Check sheet for the modelled part. Datum: model origin and axes. Units: mm. A direction names the side the tool comes from. Round coordinates to 2 decimals unless told otherwise and drop trailing zeros. Order: outer loops, then holes, each group sorted by start corner. A loop starts at its lowest first (then second) coordinate and runs counter-clockwise, first axis right, second up. Notation, with made-up numbers: (19.5, -34.5) -> (38.5, -34.5) arc R26 ccw to (38.5, -8.5) -> close; hole circle Ø3 at (76, 86). An arc over 180 degrees is marked (long way). Answer in a Markdown table with one row per item.
Autodesk Inventor part; units mm, degrees
ref_plane "YZ Plane" through (0, 0, 0) normal (1, 0, 0) x (0, 1, 0)
ref_plane "XZ Plane" through (0, 0, 0) normal (0, 1, 0) x (-1, 0, 0)
ref_plane "XY Plane" through (0, 0, 0) normal (0, 0, 1) x (1, 0, 0)
sketch "Boceto1" plane through (0, 0, 0) normal (0, 0, 1) x (1, 0, 0)
  line L0 (0, 0) -> (0, 0.3)
  line L1 (1.35, 0.9) -> (1.35, 11.3)
  line L2 (1.35, 11.3) -> (0, 0.3)
  line L3 (3.75, 0.9) -> (3.75, 11.3)
  line L4 (3.75, 11.3) -> (5.1, 0.3)
  line L5 (5.1, 0) -> (5.1, 0.3)
  line L6 (1.35, 0.9) -> (3.75, 0.9)
  line L7 (3.75, 0.6) -> (1.35, 0.6)
  line L8 (3.75, 0.6) -> (3.75, 0)
  line L9 (1.35, 0.6) -> (1.35, 0)
  line L10 (0, 0) -> (1.35, 0)
  line L11 (3.75, 0) -> (5.1, 0)
  line L12 (1.35, 11.3) -> (1.85, 11.3)
  line L13 (1.85, 11.3) -> (1.85, 0.9)
  line L14 (3.75, 11.3) -> (3.25, 11.3)
  line L15 (3.25, 11.3) -> (3.25, 0.9)
extrude "Extrusión1" add sketch "Boceto1" along normal blind 1.2 contours L0 L2 L1 L6 L3 L4 L5 L11 L8 L7 L9 L10
sketch "Boceto2" plane through (1.35, 0.9, 0) normal (0, 1, 0) x (1, 0, 0)
  line L0 (2.55, 0) -> (-0.15, 0)
  line L1 (-0.15, 0) -> (-0.15, -1.2)
  line L2 (-0.15, -1.2) -> (2.55, -1.2)
  line L3 (2.55, -1.2) -> (2.55, 0)
  line L4 (0, 0) -> (0, -1.2)
  line L5 (2.4, 0) -> (2.4, -1.2)
  line L6 (-0.15, -1.2) -> (-1.35, -1.2)
  line L7 (-1.35, -1.2) -> (-1.35, 0)
  line L8 (-1.35, 0) -> (-0.15, 0)
  line L9 (-0.15, 0) -> (-0.15, -0.15)
  line L10 (-0.15, -0.15) -> (-1.35, -0.15)
  line L11 (-1.35, -1.05) -> (-0.15, -1.05)
  line L12 (2.55, -1.2) -> (3.75, -1.2)
  line L13 (3.75, -1.2) -> (3.75, 0)
  line L14 (3.75, 0) -> (2.55, 0)
  line L15 (2.55, -0.15) -> (3.75, -0.15)
  line L16 (3.75, -1.05) -> (2.55, -1.05)
  line L17 (2.4, 0) -> (1.9, 0)
  line L18 (1.9, 0) -> (1.9, -0.15)
  line L19 (0, 0) -> (0.5, 0)
  line L20 (0.5, 0) -> (0.5, -0.15)
  arc A0 (2.3906, -1.2) -> (1.9, -0.3753) centre (1.2, -1.35) ccw
  line L21 (0, -1.2) -> (0.0094, -1.2)
  line L22 (0.5, -0.15) -> (0.5, -0.3753)
  line L23 (1.9, -0.15) -> (1.9, -0.3753)
  line L24 (2.4, -1.2) -> (2.3906, -1.2)
  arc A1 (0.5, -0.3753) -> (0.0094, -1.2) centre (1.2, -1.35) ccw
  line L25 (0, 0) -> (-1.35, 0)
  line L26 (-1.35, 0) -> (-1.35, -1.2)
  line L27 (0, -1.2) -> (-1.35, -1.2)
  line L28 (0, 0) -> (0, -1.2)
  line L29 (3.75, 0) -> (2.4, 0)
  line L30 (2.4, 0) -> (2.4, -1.2)
  line L31 (3.75, -1.2) -> (2.4, -1.2)
  line L32 (3.75, 0) -> (3.75, -1.2)
  line L33 (2.4, 0) -> (0, 0)
  line L34 (0, 0) -> (0, -1.2)
  line L35 (2.4, -1.2) -> (0, -1.2)
  line L36 (2.4, 0) -> (2.4, -1.2)
extrude "Extrusión2" cut sketch "Boceto2" along normal blind 12 contours L15 L13 L16 L3 | L1 L11 L7 L10
sketch "Boceto3" plane through (1.35, 0.9, 0) normal (0, 1, 0) x (1, 0, 0)
  line L0 (2.55, 0) -> (-0.15, 0)
  line L1 (-0.15, 0) -> (-0.15, -1.2)
  line L2 (-0.15, -1.2) -> (2.55, -1.2)
  line L3 (2.55, -1.2) -> (2.55, 0)
  line L4 (0, 0) -> (0, -1.2)
  line L5 (2.4, 0) -> (2.4, -1.2)
  line L6 (-0.15, -1.2) -> (-1.35, -1.2)
  line L7 (-1.35, -1.2) -> (-1.35, 0)
  line L8 (-1.35, 0) -> (-0.15, 0)
  line L9 (-0.15, 0) -> (-0.15, -0.15)
  line L10 (-0.15, -0.15) -> (-1.35, -0.15)
  line L11 (-1.35, -1.05) -> (-0.15, -1.05)
  line L12 (2.55, -1.2) -> (3.75, -1.2)
  line L13 (3.75, -1.2) -> (3.75, 0)
  line L14 (3.75, 0) -> (2.55, 0)
  line L15 (2.55, -0.15) -> (3.75, -0.15)
  line L16 (3.75, -1.05) -> (2.55, -1.05)
  line L17 (2.4, 0) -> (1.9, 0)
  line L18 (1.9, 0) -> (1.9, -0.15)
  line L19 (0, 0) -> (0.5, 0)
  line L20 (0.5, 0) -> (0.5, -0.15)
  arc A0 (2.3906, -1.2) -> (1.9, -0.3753) centre (1.2, -1.35) ccw
  line L21 (0, -1.2) -> (0.0094, -1.2)
  line L22 (0.5, -0.15) -> (0.5, -0.3753)
  line L23 (1.9, -0.15) -> (1.9, -0.3753)
  line L24 (2.4, -1.2) -> (2.3906, -1.2)
  arc A1 (0.5, -0.3753) -> (0.0094, -1.2) centre (1.2, -1.35) ccw
  line L25 (0, 0) -> (-1.35, 0)
  line L26 (-1.35, 0) -> (-1.35, -1.2)
  line L27 (0, -1.2) -> (-1.35, -1.2)
  line L28 (0, 0) -> (0, -1.2)
  line L29 (3.75, 0) -> (2.4, 0)
  line L30 (2.4, 0) -> (2.4, -1.2)
  line L31 (3.75, -1.2) -> (2.4, -1.2)
  line L32 (3.75, 0) -> (3.75, -1.2)
  line L33 (2.4, 0) -> (0, 0)
  line L34 (0, 0) -> (0, -1.2)
  line L35 (2.4, -1.2) -> (0, -1.2)
  line L36 (2.4, 0) -> (2.4, -1.2)
extrude "Extrusión3" add sketch "Boceto3" along normal blind 10.4 contours L5 L2 A0 L23 L18 L0 | L20 L22 A1 L2 L4 L0
sketch "Boceto4" plane through (1.35, 11.3, 0) normal (0, 1, 0) x (1, 0, 0)
  line L0 (0, 0) -> (0, -1.2)
  line L1 (0, -1.2) -> (0.0094, -1.2)
  arc A0 (0.5, -0.3753) -> (0.0094, -1.2) centre (1.2, -1.35) ccw
  line L2 (0.5, -0.3753) -> (0.5, 0)
  line L3 (0.5, 0) -> (0, 0)
  line L4 (2.4, 0) -> (1.9, 0)
  line L5 (1.9, 0) -> (1.9, -0.3753)
  arc A1 (2.3906, -1.2) -> (1.9, -0.3753) centre (1.2, -1.35) ccw
  line L6 (2.3906, -1.2) -> (2.4, -1.2)
  line L7 (2.4, 0) -> (2.4, -1.2)
  line L8 (2.55, 0) -> (-0.15, 0)
  line L9 (-0.15, 0) -> (-0.15, -1.2)
  line L10 (-0.15, -1.2) -> (2.55, -1.2)
  line L11 (2.55, -1.2) -> (2.55, 0)
  line L12 (0, 0) -> (0, -1.2)
  line L13 (2.4, 0) -> (2.4, -1.2)
  line L14 (-0.15, -1.2) -> (-1.35, -1.2)
  line L15 (-1.35, -1.2) -> (-1.35, 0)
  line L16 (-1.35, 0) -> (-0.15, 0)
  line L17 (-0.15, 0) -> (-0.15, -0.15)
  line L18 (-0.15, -0.15) -> (-1.35, -0.15)
  line L19 (-1.35, -1.05) -> (-0.15, -1.05)
  line L20 (2.55, -1.2) -> (3.75, -1.2)
  line L21 (3.75, -1.2) -> (3.75, 0)
  line L22 (3.75, 0) -> (2.55, 0)
  line L23 (2.55, -0.15) -> (3.75, -0.15)
  line L24 (3.75, -1.05) -> (2.55, -1.05)
  line L25 (2.4, 0) -> (1.9, 0)
  line L26 (1.9, 0) -> (1.9, -0.15)
  line L27 (0, 0) -> (0.5, 0)
  line L28 (0.5, 0) -> (0.5, -0.15)
  arc A2 (2.3906, -1.2) -> (1.9, -0.3753) centre (1.2, -1.35) ccw
  line L29 (0, -1.2) -> (0.0094, -1.2)
  line L30 (0.5, -0.15) -> (0.5, -0.3753)
  line L31 (1.9, -0.15) -> (1.9, -0.3753)
  line L32 (2.4, -1.2) -> (2.3906, -1.2)
  arc A3 (0.5, -0.3753) -> (0.0094, -1.2) centre (1.2, -1.35) ccw
  point P0 (-1.35, 0)
extrude "Extrusión4" add sketch "Boceto4" against normal blind 10.4 contours L0 L10 L9 L8 | L8 L11 L10 L7
sketch "Boceto5" plane through (1.35, 11.3, 0) normal (0, 1, 0) x (1, 0, 0)
  line L0 (2.55, 0) -> (-0.15, 0)
  line L1 (-0.15, 0) -> (-0.15, -1.2)
  line L2 (-0.15, -1.2) -> (2.55, -1.2)
  line L3 (0, 0) -> (0, -1.2)
  line L4 (2.4, 0) -> (2.4, -1.2)
  line L5 (0, -1.2) -> (0.0094, -1.2)
  line L6 (0.5, -0.15) -> (0.5, -0.3753)
  line L7 (0, 0) -> (0.5, 0)
  line L8 (0.5, 0) -> (0.5, -0.15)
  arc A0 (0.5, -0.3753) -> (0.0094, -1.2) centre (1.2, -1.35) ccw
  line L9 (2.4, -1.2) -> (0, -1.2)
  line L10 (2.4, 0) -> (0, 0)
  line L11 (1.9, 0) -> (1.9, -0.15)
  line L12 (2.4, 0) -> (1.9, 0)
  line L13 (-0.15, -1.2) -> (-1.35, -1.2)
  line L14 (-1.35, -1.2) -> (-1.35, 0)
  line L15 (-1.35, 0) -> (-0.15, 0)
  line L16 (-0.15, 0) -> (-0.15, -0.15)
  line L17 (0, 0) -> (0, -1.2)
  line L18 (0, 0) -> (-1.35, 0)
  line L19 (-0.15, -0.15) -> (-1.35, -0.15)
  line L20 (-1.35, -1.05) -> (-0.15, -1.05)
  line L21 (-1.35, 0) -> (-1.35, -1.2)
  line L22 (0, -1.2) -> (-1.35, -1.2)
  line L23 (0, 0) -> (0, -1.2)
  line L24 (2.55, -1.2) -> (2.55, 0)
  line L25 (2.55, -1.2) -> (3.75, -1.2)
  line L26 (3.75, -1.2) -> (3.75, 0)
  line L27 (3.75, 0) -> (2.55, 0)
  line L28 (2.55, -0.15) -> (3.75, -0.15)
  line L29 (3.75, -1.05) -> (2.55, -1.05)
  line L30 (1.9, -0.15) -> (1.9, -0.3753)
  arc A1 (2.3906, -1.2) -> (1.9, -0.3753) centre (1.2, -1.35) ccw
  line L31 (2.4, -1.2) -> (2.3906, -1.2)
  line L32 (2.4, 0) -> (2.4, -1.2)
  line L33 (2.4, 0) -> (2.4, -1.2)
  line L34 (3.75, -1.2) -> (2.4, -1.2)
  line L35 (3.75, 0) -> (3.75, -1.2)
  line L36 (3.75, 0) -> (2.4, 0)
extrude "Extrusión5" cut sketch "Boceto5" against normal blind 11 contours L28 L26 L29 L24 | L1 L20 L14 L19
sketch "Boceto6" plane through (1.35, 0.3, 0) normal (0, 1, 0) x (1, 0, 0)
  line L0 (2.55, 0) -> (-0.15, 0)
  line L1 (-0.15, 0) -> (-0.15, -1.2)
  line L2 (-0.15, -1.2) -> (2.55, -1.2)
  line L3 (2.55, -1.2) -> (2.55, 0)
  line L4 (0, 0) -> (0, -1.2)
  line L5 (2.4, 0) -> (2.4, -1.2)
  line L6 (-0.15, -1.2) -> (-1.35, -1.2)
  line L7 (-1.35, -1.2) -> (-1.35, 0)
  line L8 (-1.35, 0) -> (-0.15, 0)
  line L9 (-0.15, 0) -> (-0.15, -0.15)
  line L10 (-0.15, -0.15) -> (-1.35, -0.15)
  line L11 (-1.35, -1.05) -> (-0.15, -1.05)
  line L12 (2.55, -1.2) -> (3.75, -1.2)
  line L13 (3.75, -1.2) -> (3.75, 0)
  line L14 (3.75, 0) -> (2.55, 0)
  line L15 (2.55, -0.15) -> (3.75, -0.15)
  line L16 (3.75, -1.05) -> (2.55, -1.05)
  line L17 (2.4, 0) -> (1.9, 0)
  line L18 (1.9, 0) -> (1.9, -0.15)
  line L19 (0, 0) -> (0.5, 0)
  line L20 (0.5, 0) -> (0.5, -0.15)
  arc A0 (2.3906, -1.2) -> (1.9, -0.3753) centre (1.2, -1.35) ccw
  line L21 (0, -1.2) -> (0.0094, -1.2)
  line L22 (0.5, -0.15) -> (0.5, -0.3753)
  line L23 (1.9, -0.15) -> (1.9, -0.3753)
  line L24 (2.4, -1.2) -> (2.3906, -1.2)
  arc A1 (0.5, -0.3753) -> (0.0094, -1.2) centre (1.2, -1.35) ccw
  circle A2 centre (2.75, -0.6) radius 0.15
  circle A3 centre (3.35, -0.6) radius 0.15
  circle A4 centre (-0.35, -0.6) radius 0.15
  circle A5 centre (-0.95, -0.6) radius 0.15
  line L25 (-1.35, 0) -> (-1.35, -0.15)
  line L26 (-1.35, -0.15) -> (-1.35, -1.05)
  line L27 (-1.35, -1.05) -> (-1.35, -1.2)
extrude "Extrusión6" cut sketch "Boceto6" against normal blind 10 contours A2 | A3 | A4 | A5
sketch "Boceto7" plane through (0, 0, 1.2) normal (0, 0, 1) x (1, 0, 0)
  line L0 (0, 0) -> (1.35, 0)
  line L1 (1.35, 0) -> (1.3594, 6.1)
  line L2 (1.3594, 0.9) -> (1.3594, 11.3)
  line L3 (1.3594, 6.1) -> (7.7947, 6.0901)
  line L4 (7.7947, 6.0901) -> (7.8047, 12.5901)
  line L5 (7.8047, 12.5901) -> (-2.1953, 12.6055)
  line L6 (-2.1953, 12.6055) -> (-2.2053, 6.1055)
  line L7 (-2.2053, 6.1055) -> (1.3594, 6.1)
  dimension "d12" = 6.1
  dimension "d13" = 6.5
  dimension "d14" = 10
extrude "Extrusión7" cut sketch "Boceto7" against normal blind 10
sketch "Boceto8" plane through (0, 0, 1.2) normal (0, 0, 1) x (1, 0, 0)
  line L0 (1.2, 6.1002) -> (1.2, 0.3)
  line L1 (3.9, 6.0961) -> (3.9, 0.3)
  line L2 (0, 0.3) -> (0, 0)
  line L3 (5.1, 0) -> (5.1, 0.3)
  line L4 (0, 0.3) -> (1.2, 6.1002)
  line L5 (1.2, 6.873) -> (1.2, 6.1002)
  line L6 (0, 0.3) -> (-0.3806, 0.3)
  line L7 (-0.3806, 0.3) -> (-0.3806, 6.873)
  line L8 (-0.3806, 6.873) -> (1.2, 6.873)
  line L9 (3.25, 0.9) -> (1.85, 0.9)
  line L10 (2.55, 0.9) -> (2.55, 4.8471)
  line L11 (3.9, 6.1002) -> (3.9, 0.3)
  line L12 (5.1, 0.3) -> (5.1, 0)
  line L13 (5.1, 0.3) -> (3.9, 6.1002)
  line L14 (3.9, 6.873) -> (3.9, 6.1002)
  line L15 (5.1, 0.3) -> (5.4806, 0.3)
  line L16 (5.4806, 0.3) -> (5.4806, 6.873)
  line L17 (5.4806, 6.873) -> (3.9, 6.873)
extrude "Extrusión8" cut sketch "Boceto8" against normal blind 10
sketch "Boceto9" plane through (0, 0, 1.2) normal (0, 0, 1) x (1, 0, 0)
  line L0 (0, 0) -> (0, 0.3)
  line L1 (1.35, 0.9) -> (1.35, 6.1)
  line L2 (1.2, 6.1) -> (0, 0.3)
  line L3 (3.75, 0.9) -> (3.75, 6.1)
  line L4 (3.9, 6.1) -> (5.1, 0.3)
  line L5 (5.1, 0) -> (5.1, 0.3)
  line L6 (1.35, 0.9) -> (3.75, 0.9)
  line L7 (3.75, 0.6) -> (1.35, 0.6)
  line L8 (3.75, 0.6) -> (3.75, 0)
  line L9 (1.35, 0.6) -> (1.35, 0)
  line L10 (0, 0) -> (1.35, 0)
  line L11 (3.75, 0) -> (5.1, 0)
  line L12 (1.85, 6.1) -> (1.85, 0.9)
  line L13 (3.25, 6.1) -> (3.25, 0.9)
  line L14 (1.2, 6.1) -> (1.85, 6.1)
  line L15 (3.25, 6.1) -> (3.75, 6.1)
  line L16 (1.35, 6.1) -> (1.2, 6.1)
  line L17 (3.75, 6.1) -> (3.9, 6.1)
  circle A0 centre (1.0336, 4) radius 0.15
  circle A1 centre (1.0336, 3.1) radius 0.15
  circle A2 centre (4.0664, 4) radius 0.15
  circle A3 centre (4.0664, 3.1) radius 0.15
  line L18 (1.35, 0.6) -> (3.75, 0.6)
  point P0 (0, 0)
extrude "Extrusión9" cut sketch "Boceto9" against normal blind 0.5 contours A0 | A1 | A2 | A3
properties part number "learnbotEncajeBateria"
(1) Section check D-D on x = 1.05. Record the boundary of the cut face in (y, z).
Solutions:
| item | result |
|---|---|
| outline | (0, 0) -> (5.38, 0) -> (5.38, 0.15) -> (0.3, 0.15) -> (0.3, 0.46) -> (0, 0.46) -> close; (0, 0.74) -> (0.3, 0.74) -> (0.3, 1.05) -> (2.95, 1.05) -> (2.95, 1.2) -> (0, 1.2) -> close; (3.25, 1.05) -> (3.85, 1.05) -> (3.85, 1.2) -> (3.25, 1.2) -> close; (4.15, 1.05) -> (5.38, 1.05) -> (5.38, 1.2) -> (4.15, 1.2) -> close |
(2) Draft check along Z on faces 1 (the flat face through (3, 0.9, 1)), 2 (the flat face through (3.9, 3.2, 0.6)), 3 (the flat face through (3.6, 2.4, 0)), 4 (the flat face through (4.4, 0.3, 0.7)). Enter one of: pulls with the +Z half, pulls with the -Z half, needs draft (parallel to the pull), parting line crosses it, or undercut.
Solutions:
| item | result |
|---|---|
| face 1 | needs draft |
| face 2 | undercut |
| face 3 | pulls with the -Z half |
| face 4 | undercut |
(3) Tool access check on faces 5 (the flat face through (0.7, 0.3, 0.7)), 6 (the cylindrical face through (1.515, 3.464, 0.742)), 7 (the flat face through (3, 0.6, 1)). Record the directions out of +Z, -Z, +X, -X, +Y, -Y that give a thin tool (end or side, any length) a straight path to the whole face; none if there is none.
Solutions:
| item | result |
|---|---|
| face 5 | -X, +Y |
| face 6 | +Z, +Y |
| face 7 | +Z, -Z, -Y |
(4) Section check B-B on x = 4.7. Record the boundary of the cut face in (y, z), plus the area to 3 significant figures.
Solutions:
| item | result |
|---|---|
| outline | (0, 0) -> (2.23, 0) -> (2.23, 0.15) -> (0.3, 0.15) -> (0.3, 0.45) -> (0, 0.45) -> close; (0, 0.75) -> (0.3, 0.75) -> (0.3, 1.05) -> (2.23, 1.05) -> (2.23, 1.2) -> (0, 1.2) -> close |
| area | 0.850 mm^2 |
(5) Section check A-A on y = 2.75. Record the boundary of the cut face in (x, z), plus the area to 3 significant figures.
Solutions:
| item | result |
|---|---|
| outline | (0.51, 0) -> (1.85, 0) -> (1.85, 0.38) arc R1.2 cw to (1.36, 1.2) -> (0.51, 1.2) -> (0.51, 1.05) -> (1.2, 1.05) -> (1.2, 0.15) -> (0.51, 0.15) -> close; (3.25, 0) -> (4.59, 0) -> (4.59, 0.15) -> (3.9, 0.15) -> (3.9, 1.05) -> (4.59, 1.05) -> (4.59, 1.2) -> (3.74, 1.2) arc R1.2 cw to (3.25, 0.38) -> close |
| area | 1.44 mm^2 |
(6) Scan lines: probe 1 along X at (y, z) = (0.1, 0.6); probe 2 along Z at (x, y) = (0.4, 0.25); probe 3 along Y at (x, z) = (3.4, 1.15). Record each from-to range of solid material in increasing order. Write a range as from..to.
Solutions:
| item | result |
|---|---|
| probe 1 | 0..0.25, 0.55..0.85, 1.15..1.35, 3.75..3.95, 4.25..4.55, 4.85..5.1 |
| probe 2 | 0..0.45, 0.75..1.2 |
| probe 3 | 0.6..0.9 |
(7) Depth check by flat-ended pin: pin 1 Ø0.6 at (x, z) = (2.5, 0.5) entering from +Y; pin 2 Ø1 at (x, y) = (1.5, 1.5) entering from +Z; pin 3 Ø0.5 at (x, z) = (4.5, 0.5) entering from +Y; pin 4 Ø0.5 at (y, z) = (4.5, 0.5) entering from +X. Enter the tip coordinate at first touch or a pass-through.
Solutions:
| item | result |
|---|---|
| pin 1 | y = 0.9 |
| pin 2 | z = 1.2 |
| pin 3 | y = 0.3 |
| pin 4 | x = 3.9 |
(8) Section check C-C on z = 0.25. Record the boundary of the cut face in (x, y).
Solutions:
| item | result |
|---|---|
| outline | (0, 0) -> (1.35, 0) -> (1.35, 0.6) -> (3.75, 0.6) -> (3.75, 0) -> (5.1, 0) -> (5.1, 0.3) -> (3.9, 0.3) -> (3.9, 6.1) -> (3.25, 6.1) -> (3.25, 0.9) -> (1.85, 0.9) -> (1.85, 6.1) -> (1.36, 6.1) -> (1.2, 6.1) -> (1.2, 0.3) -> (0, 0.3) -> close |
